Could you check a few things on this model? Use its own coordinates, in mm. A direction names the side the tool comes from. Give positions to 0.01 mm unless a question says otherwise; leave off trailing zeros. Order: outer loops, then holes, each group sorted by start corner. A loop starts at its lowest first (then second) coordinate and runs counter-clockwise, first axis right, second up. Notation, with made-up numbers: (-2, 63) - (27, 63) arc R15 cw to (27, 92) - close; hole circle Ø8 at (-6, -33). An arc over 180 degrees is marked (long way). Put each result on its own line as item: value.
Autodesk Inventor part; units mm, degrees
ref_plane "YZ Plane" through (0, 0, 0) normal (1, 0, 0) x (0, 1, 0)
ref_plane "XY Plane" through (0, 0, 0) normal (0, 0, 1) x (1, 0, 0)
sketch "Sketch1" plane through (0, 0, 0) normal (0, 0, 1) x (1, 0, 0)
  circle A0 centre (0, 0) radius 142.875
  circle A1 centre (0, 0) radius 149.225
  dimension "innerDiameter" = 285.75
  dimension "outerDiameter" = 298.45
extrude "Extrusion1" add sketch "Sketch1" along normal mid plane 19.05
sketch "Sketch2" plane through (0, 0, 0) normal (0, 0, 1) x (1, 0, 0)
  circle A0 centre (0, 0) radius 142.875 construction
  line L0 (0, 142.875) -> (0, 149.225) construction
  circle A1 centre (0, 0) radius 149.225 construction
  line L1 (0, 142.875) -> (44.45, 142.875)
  line L2 (44.45, 142.875) -> (44.45, 149.225)
  line L3 (44.45, 149.225) -> (19.05, 149.225)
  line L4 (0, 142.875) -> (-44.45, 142.875)
  line L5 (-44.45, 142.875) -> (-44.45, 149.225)
  line L6 (-44.45, 149.225) -> (19.05, 149.225)
  line L7 (371.6693, 35.081) -> (0, 0)
  dimension "halfBaseWidth" = 44.45
  dimension "baseThickness" = 6.35
  dimension "baseHeight" = 0
extrude "Extrusion2" add sketch "Sketch2" along normal mid plane 19.05
sketch "Sketch5" plane through (-44.45, 149.225, 9.525) normal (0, 1, 0) x (1, 0, 0)
  line L0 (0, 19.05) -> (0, 0)
  line L1 (88.9, 19.05) -> (88.9, 0)
  line L2 (0, 0) -> (88.9, 0)
  line L3 (88.9, 0) -> (88.9, 19.05)
  line L4 (88.9, 19.05) -> (0, 19.05)
  line L5 (0, 19.05) -> (0, 0)
  point P0 (44.45, 9.525)
  point P1 (0, 19.05)
extrude "Extrusion3" add sketch "Sketch5" along normal blind 63.5
sketch "Sketch7" plane through (0, 0, 9.525) normal (0, 0, 1) x (1, 0, 0)
  line L0 (-44.45, 142.875) -> (-44.45, 212.725)
  line L1 (-44.45, 212.725) -> (44.45, 212.725)
  line L2 (44.45, 142.875) -> (44.45, 212.725)
  line L3 (0, 212.725) -> (0, 149.1868) construction
  line L4 (-15.875, 197.104) -> (15.875, 197.104)
  line L5 (15.875, 197.104) -> (15.875, 206.375)
  line L6 (15.875, 206.375) -> (-15.875, 206.375)
  line L7 (-15.875, 206.375) -> (-15.875, 197.104)
  line L8 (-15.875, 197.104) -> (15.875, 206.375) construction
  line L9 (15.875, 197.104) -> (-15.875, 206.375) construction
  point P0 (0, 0)
  point P1 (-38.1, 144.2792)
  point P2 (38.1, 144.2792)
  point P3 (0, 201.7395)
  dimension "screwHoleWidth" = 31.75
  dimension "screwHoleHeight" = 9.271
  dimension "screwHoleSupportThickness" = 6.35
extrude "Extrusion4" cut sketch "Sketch7" against normal through all
sketch "Sketch6" plane through (-44.45, 212.725, 9.525) normal (0, 1, 0) x (1, 0, 0)
  point P0 (44.45, 9.525)
  point P1 (44.45, 9.525)
hole "Hole2" at (0, 212.725, 0) direction (0, -1, 0) diameter 6.7564 depth 6.35
ref_plane "Work Plane1" through (0, 0, 0) normal (-0.7071, 0.7071, 0) x (0, 0, 1)
ref_plane "Work Plane2" through (0, 0, 0) normal (0.7071, 0.7071, 0) x (0, 0, 1)
sketch "Sketch11" plane through (0, 0, 0) normal (0, 0, 1) x (1, 0, 0)
  arc A0 (-43.0678, 142.875) -> (43.0678, 142.875) centre (0, 0) ccw
  circle A1 centre (0, 0) radius 142.875
  line L0 (-214.9625, 214.9625) -> (217.3313, -217.3313)
  line L1 (-101.0279, 101.0279) -> (-96.5378, 105.518)
  line L2 (-101.0279, 101.0279) -> (-94.6779, 101.0279) construction
  line L3 (-96.5378, 105.518) -> (-114.4983, 123.4785)
  line L4 (-96.5378, 105.518) -> (-71.1378, 105.518) construction
  line L5 (-114.4983, 123.4785) -> (-118.9884, 118.9884)
  line L6 (-118.9884, 118.9884) -> (-101.0279, 101.0279)
  line L7 (-101.0279, 101.0279) -> (-105.518, 96.5378)
  line L8 (-105.518, 96.5378) -> (-123.4785, 114.4983)
  line L9 (-123.4785, 114.4983) -> (-118.9884, 118.9884)
  point P0 (38.1, 144.2792)
  point P1 (-38.1, 144.2792)
  point P2 (-109.9126, 100.9323)
  point P3 (-100.9323, 109.9126)
  dimension "d47" = 6.35
  dimension "d48" = 45
  dimension "d49" = 25.4
  dimension "d50" = 135
extrude "Extrusion7" add sketch "Sketch11" along normal mid plane 19.05 contours A0 L0 L5 L3 | A0 L8 L9 L0
sketch "Sketch12" plane through (-114.4983, 123.4785, -9.525) normal (0.7071, 0.7071, 0) x (-0.7071, 0.7071, 0)
  line L0 (0, 0) -> (0, 19.05)
  line L1 (-19.1852, 19.05) -> (0, 19.05)
  line L2 (-19.1852, 0) -> (-19.1852, 19.05)
  line L3 (0, 0) -> (-19.1852, 0)
  line L4 (-9.5926, 19.05) -> (-9.5926, 0) construction
  line L5 (0, 9.525) -> (-19.1852, 9.525) construction
  point P0 (-168.275, 9.525)
  point P1 (-9.5926, 9.525)
hole "Hole4" at (-107.7153, 116.6955, 0) direction (-0.7071, -0.7071, 0) diameter 5.1054 depth 12.7
pattern_circular "Circular Pattern1" count 4 over 360 about axis through (0, 0, -10) along (0, 0, 1) of "Extrusion7", "Hole4"
sketch "Sketch13" plane through (0, 0, 9.525) normal (0, 0, 1) x (1, 0, 0)
  line L0 (-15.875, 206.375) -> (15.875, 206.375)
  line L1 (-44.45, 212.725) -> (44.45, 212.725)
  line L2 (0, 208.915) -> (8.89, 208.915)
  line L3 (8.89, 208.915) -> (8.89, 206.375)
  line L4 (8.89, 206.375) -> (0, 206.375)
  line L5 (0, 208.915) -> (0, 206.375)
  line L6 (15.875, 206.375) -> (-15.875, 206.375)
  line L7 (0, 208.915) -> (-8.89, 208.915)
  line L8 (-8.89, 208.915) -> (-8.89, 206.375)
  point P0 (0, 0)
  dimension "d63" = 8.89
  dimension "d64" = 2.54
extrude "Extrusion8" cut sketch "Sketch13" against normal through all
sketch "Sketch14" plane through (0, 0, 9.525) normal (0, 0, 1) x (1, 0, 0)
  point P0 (0, 0)
sketch "Sketch15" plane through (0, 0, 0) normal (0, 0, 1) x (1, 0, 0)
  arc A0 (-43.0678, 142.875) -> (-100.9323, 109.9126) centre (0, 0) ccw
  line L0 (-43.0678, 142.875) -> (-44.45, 142.875)
  line L1 (44.45, 142.875) -> (43.0678, 142.875)
  arc A1 (100.9323, 109.9126) -> (43.0678, 142.875) centre (0, 0) ccw
  line L2 (-44.45, 142.875) -> (-44.45, 142.451)
  line L3 (-44.45, 142.875) -> (-43.0678, 142.875)
  line L4 (43.0678, 142.875) -> (44.45, 142.875)
  line L5 (44.45, 142.875) -> (44.45, 142.451)
  arc A2 (-43.0678, 142.875) -> (-44.45, 142.451) centre (0, 0) ccw
  arc A3 (44.45, 142.451) -> (43.0678, 142.875) centre (0, 0) ccw
extrude "Extrusion9" add sketch "Sketch15" along normal mid plane 19.05
sketch "Sketch16" plane through (0, 0, 0) normal (0, 0, 1) x (1, 0, 0)
  line L0 (44.45, 142.451) -> (44.45, 212.725)
  line L1 (-44.45, 142.451) -> (-44.45, 212.725)
  arc A0 (-44.45, 142.451) -> (-100.9323, 109.9126) centre (0, 0) ccw
  arc A1 (100.9323, 109.9126) -> (44.45, 142.451) centre (0, 0) ccw
  line L2 (0, 0) -> (-74.6125, 129.2326) construction
  line L3 (0, 0) -> (0, 149.225) construction
  line L4 (0, 0) -> (74.6125, 129.2326) construction
  line L5 (-44.45, 212.725) -> (-74.6125, 129.2326)
  line L6 (-44.45, 142.451) -> (-44.45, 212.725)
  line L7 (-44.45, 142.451) -> (-44.45, 212.725)
  line L8 (44.45, 212.725) -> (44.45, 142.451)
  line L9 (44.45, 212.725) -> (74.6125, 129.2326)
  arc A2 (74.6125, 129.2326) -> (44.45, 142.451) centre (0, 0) ccw
  arc A3 (-44.45, 142.451) -> (-74.6125, 129.2326) centre (0, 0) ccw
  dimension "d69" = 30
  dimension "d70" = 30
extrude "Extrusion10" add sketch "Sketch16" along normal mid plane 19.05
fillet "Fillet1" radius 3.175 2 edges at (-74.6125, 129.2326, 0) (74.6125, 129.2326, 0)
fillet "Fillet2" radius 3.175 2 edges at (-44.45, 212.725, 0) (44.45, 212.725, 0)
split "Split3" plane through (0, 0, 0) removes the side toward (-0.7071, -0.7071, 0)
split "Split4" plane through (0, 0, 0) removes the side toward (0.7071, -0.7071, 0)
equation "\"outerDiameter\" = innerDiameter + 2 * ringThicknessRadius"
equation "\"d7\" = ringWidth"
equation "\"d51\" = ringWidth"
equation "\"d67\" = ringWidth"
equation "\"d71\" = ringWidth"
equation "\"ringThicknessRadius\" = 6.35"
properties part number "mountFirstQuater" material "PET Plastic"
1) Suppose I cut it at C-C, the plane z = 0. State how many separate pieces and enclosed holes the cut face has, and give its area (3 significant figures).
Filled in:
separate pieces: 3
enclosed holes: 0
area: 9,190 mm^2
2) We'd pull the mould along X, two halves only. Please class faces 1 (the flat face through (-1, 212.725, -4)), 2 (the cylindrical face through (2.056, 210.793, -2.681)), 3 (the flat face through (-116.712, 121.265, -0.133)): pulls with the +X half, pulls with the -X half, needs draft (parallel to the pull), parting line crosses it, or undercut.
Filled in:
face 1: needs draft
face 2: undercut
face 3: pulls with the -X half
3) Suppose I cut it at A-A, the plane x = 0. List the corners of the cut face in (y, z) for me (3 decimals).
Filled in:
outline: (142.875, -9.525) - (197.104, -9.525) - (197.104, 9.525) - (142.875, 9.525) - close; (208.915, -9.525) - (212.725, -9.525) - (212.725, -3.378) - (208.915, -3.378) - close; (208.915, 3.378) - (212.725, 3.378) - (212.725, 9.525) - (208.915, 9.525) - close
4) I'm going to push flat-ended pins straight in: pin 1 (6 mm diameter, centred on y = 163, z = 2.5, fed in from -X); pin 2 (7.5 mm diameter, centred on x = -11.5, z = 0, fed in from -Y); pin 3 (8 mm diameter, centred on x = -73, z = 2.5, fed in from -Y). Where does each tip first touch, or does it pass through?
Filled in:
pin 1: stops at x = -63.5
pin 2: stops at y = 142.06
pin 3: stops at y = 120.35
5) Which directions (+Z, -Z, +X, -X, +Y, -Y) give clear straight access to the entire face, cutting with the end or side of a thin tool? Please do faces 4 (the cylindrical face through (-1.571, 142.866, -0.133)), 5 (the cylindrical face through (88.58, 120.09, -0.13)), 6 (the flat face through (15.875, 202, 0)).
Filled in:
face 4: +Z, -Z, -Y
face 5: +Z, -Z, +Y
face 6: +Z, -Z
6) Suppose I cut it at D-D, the plane x = 37. List the corners of the cut face in (y, z) for me (3 decimals), and give its area (3 significant figures).
Filled in:
outline: (138.001, -9.525) - (212.725, -9.525) - (212.725, 9.525) - (138.001, 9.525) - close
area: 1,420 mm^2
7) Suppose I cut it at B-B, the plane y = 157. List the corners of the cut face in (x, z) for me (3 decimals), and give its area (3 significant figures).
Filled in:
outline: (-64.581, -9.525) - (64.581, -9.525) - (64.581, 9.525) - (-64.581, 9.525) - close
area: 2,460 mm^2
8) If I drill on line 1 (Z direction, x = 0, y = 210) (3 decimals); line 2 (Y direction, x = -4.5, z = 5.75) (3 decimals); line 3 (Y direction, x = 0, z = 3.5) (3 decimals), over which ranges is the centre line in solid material (lowest first)? Write a range as [from, to].
Filled in:
line 1: z = [-9.525, -3.378], [3.378, 9.525]
line 2: y = [142.804, 197.104], [208.915, 212.725]
line 3: y = [142.875, 197.104], [208.915, 212.725]
